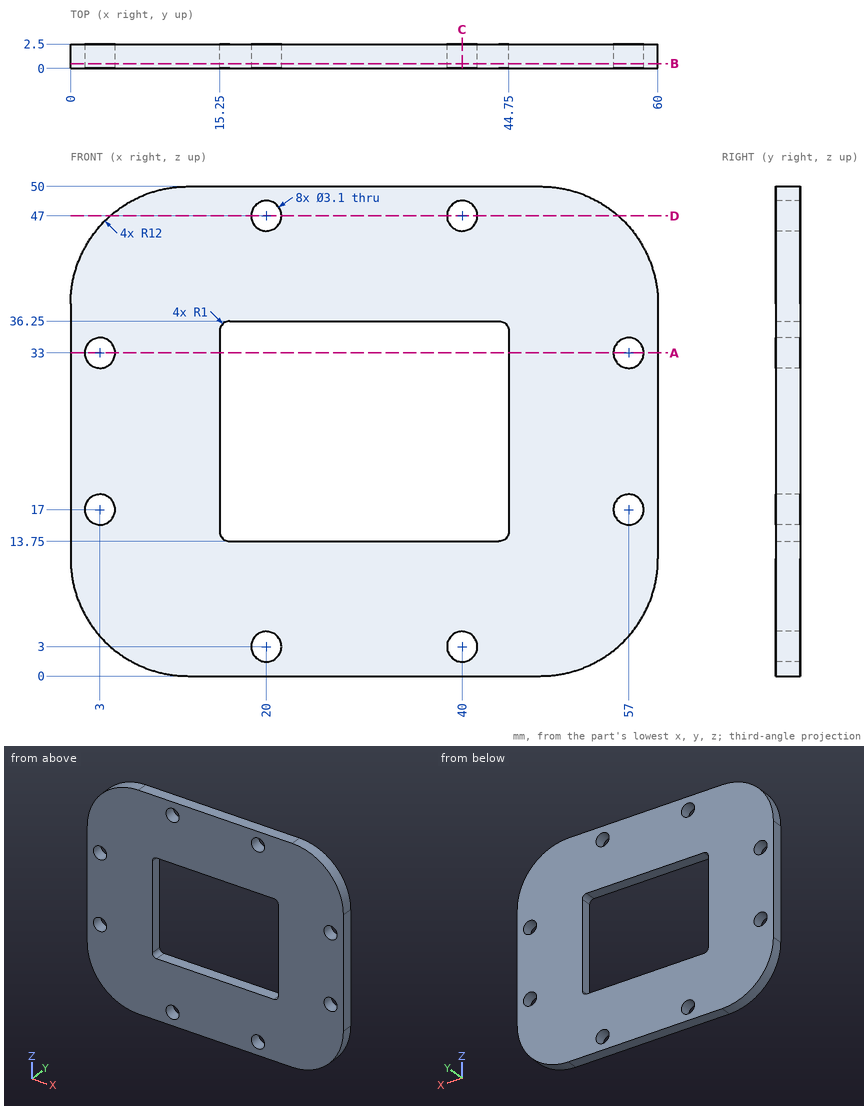
Study the drawing (mm; zero at the part's minimum x, y, z) and answer. Coordinates: 2 decimals unless noted, no trailing zeros. Loops run counter-clockwise (first coordinate to the right, second up) from the corner with the lowest first, then second, coordinate; pieces in that order, holes last. Notation, with made-up numbers: (37.25, 84) -> (93.25, 84) arc R19 cw to (93.25, 102) -> close; hole circle Ø4 at (-17.5, 18). An arc over 180 degrees is marked (long way). Write each question's results on one line, items separated by ' | '. Start each with the question number.
1) Find section C-C on x = 40. Determine the outline of the cut face in (y, z), then the cut area to 4 significant figures.
2) Find section A-A on z = 33. Determine the outline of the cut face in (x, y).
3) Find section B-B on y = 0.5. Count the separate pieces of the cut face and the enclosed holes in it, then the cut area to 3 significant figures.
4) Consider line 1 along Z through (x, y) = (40, 1.1); line 2 along Z through (x, y) = (26.5, 1.3); line 3 along X through (y, z) = (1.75, 21). Determine where each line is inside the solid, lowest interval first.
5) Find section D-D on z = 47. Determine the outline of the cut face in (x, y).
6) Flat-ended cylindrical pins translate along their axes: P1, Ø3, axis at x = 57, z = 17, coming from the -Y side; P2, Ø3, axis at x = 35, z = 8.5, coming from the -Y side. Find the tip coordinate at first contact, or state that the pin passes through.
Response values:
1) outline: (0, 0) -> (2.5, 0) -> (2.5, 1.45) -> (0, 1.45) -> close; (0, 4.55) -> (2.5, 4.55) -> (2.5, 13.75) -> (0, 13.75) -> close; (0, 36.25) -> (2.5, 36.25) -> (2.5, 45.45) -> (0, 45.45) -> close; (0, 48.55) -> (2.5, 48.55) -> (2.5, 50) -> (0, 50) -> close | area: 53.25 mm^2
2) outline: (0, 0) -> (1.45, 0) -> (1.45, 2.5) -> (0, 2.5) -> close; (4.55, 0) -> (15.25, 0) -> (15.25, 2.5) -> (4.55, 2.5) -> close; (44.75, 0) -> (55.45, 0) -> (55.45, 2.5) -> (44.75, 2.5) -> close; (58.55, 0) -> (60, 0) -> (60, 2.5) -> (58.55, 2.5) -> close
3) separate pieces: 1 | enclosed holes: 9 | area: 2,150 mm^2
4) line 1: z = 0 to 1.45, 4.55 to 13.75, 36.25 to 45.45, 48.55 to 50 | line 2: z = 0 to 13.75, 36.25 to 50 | line 3: x = 0 to 15.25, 44.75 to 60
5) outline: (4.06, 0) -> (18.45, 0) -> (18.45, 2.5) -> (4.06, 2.5) -> close; (21.55, 0) -> (38.45, 0) -> (38.45, 2.5) -> (21.55, 2.5) -> close; (41.55, 0) -> (55.94, 0) -> (55.94, 2.5) -> (41.55, 2.5) -> close
6) P1: passes through | P2: stops at y = 0
